```python
from build123d import *

# Parameters (mm, degrees)
SKETCH_1_R      = 4
SKETCH_1_R_2    = 2
EXTRUDE_1_DEPTH = 2
SKETCH_2_R      = 4
SKETCH_2_R_2    = 2
EXTRUDE_2_DEPTH = 2
FILLET_1_R      = 2


with BuildPart() as part:
    # 草图1 → 凸台-拉伸1 (new body)
    with BuildSketch(Plane(origin=(0, 0, 0), x_dir=(1, 0, 0), z_dir=(0, 1, 0))):
        with BuildLine():
            Line((-11.25, 12.5), (11.25, 12.5))
            ThreePointArc((11.25, 12.5), (23.75, 0), (11.25, -12.5))
            Line((11.25, -12.5), (-11.25, -12.5))
            Line((-11.25, -12.5), (-11.25, 12.5))
        make_face()
        with Locations((11.25, 0)):
            Circle(SKETCH_1_R, mode=Mode.SUBTRACT)
        with Locations((18.25, 0)):
            Circle(SKETCH_1_R_2, mode=Mode.SUBTRACT)
        with Locations((11.25, -7)):
            Circle(SKETCH_1_R_2, mode=Mode.SUBTRACT)
        with Locations((4.25, 0)):
            Circle(SKETCH_1_R_2, mode=Mode.SUBTRACT)
        with Locations((11.25, 7)):
            Circle(SKETCH_1_R_2, mode=Mode.SUBTRACT)
    extrude(amount=EXTRUDE_1_DEPTH)

    # 草图2 → 凸台-拉伸2 (add)
    with BuildSketch(Plane.ZY.offset(11.25)):
        with BuildLine():
            Line((-12.5, 0), (12.5, 0))
            Line((12.5, 0), (12.5, 12.5))
            ThreePointArc((12.5, 12.5), (0, 25), (-12.5, 12.5))
            Line((-12.5, 12.5), (-12.5, 0))
        make_face()
        with Locations((0, 12.5)):
            Circle(SKETCH_2_R, mode=Mode.SUBTRACT)
        with Locations((0, 19.5)):
            Circle(SKETCH_2_R_2, mode=Mode.SUBTRACT)
        with Locations((7, 12.5)):
            Circle(SKETCH_2_R_2, mode=Mode.SUBTRACT)
        with Locations((0, 5.5)):
            Circle(SKETCH_2_R_2, mode=Mode.SUBTRACT)
        with Locations((-7, 12.5)):
            Circle(SKETCH_2_R_2, mode=Mode.SUBTRACT)
    extrude(amount=-EXTRUDE_2_DEPTH)

    # 圆角1
    fillet_1_edges = [part.edges().sort_by_distance(p)[0] for p in [
        (-11.25, 0, 0),
    ]]
    fillet(fillet_1_edges, radius=FILLET_1_R)


solid = part.part
```
Check sheet for the modelled part. Datum: model origin and axes. Units: mm. A direction names the side the tool comes from. Coordinates: 2 decimals unless noted, no trailing zeros. Order: outer loops, then holes, each group sorted by start corner. A loop starts at its lowest first (then second) coordinate and runs counter-clockwise, first axis right, second up. Notation, with made-up numbers: M 57,17 L 113,17 A12 ccw 113,29 Z; hole C 46.25,44.25 d4. An arc over 180 degrees is marked long. Write each question's results on one line, items separated by ' | '. Start each with the question number.
1. Cross-section at D-D on z = 9.5. Record the cut outline in (x, y), and give its area (3 significant figures).
2. Mould release check, pull along Y, two halves, no side actions. Record for faces 1 (the face through (-10.65, 0.57, -0.18)), 2 (the face through (9.252, 0.986, 6.912)), 3 (the face through (-10, 25, 0)), 4 (the face through (-10.264, 16.466, -0.521)): +Y half, -Y half, draft (parallel to the pull), parting line (faces both ways), or undercut.
3. Go/stop test with flat-tipped pins: P1, Ø6.5, axis at x = 11.25, z = -7, coming from the +Y side; P2, Ø1, axis at y = 14, z = 10, coming from the +X side; P3, Ø5, axis at x = -7, z = -4, coming from the +Y side. Record where each tip stops, or that it passes through.
4. Access from +Z, -Z, +X, -X, +Y, -Y to the whole of each face (thin tool, end or side, straight path). Record for faces 5 (the face through (4, 2, -3)), 6 (the face through (-2.4, 1.6, 12.5)).
5. Cross-section at A-A on x = 4.25. Record the cut outline in (y, z), and give its area (3 significant figures).
6. Cross-section at C-C on z = 0. State how many separate pieces and enclosed holes the cut face has, and give its area (3 significant figures).
7. Cross-section at B-B on y = 5.5. Record the cut outline in (x, z).
8. Material ranges on probe 1 along Z at (x, y) = (11.25, 0.6); probe 2 along X at (y, z) = (0.6, 0); probe 3 along Y at (x, z) = (-10.35, 0), recorded low to high.
Checks:
1) outline: M -11.25,2 A2 ccw -9.25,0 L 19.37,0 L 19.37,2 L -9.25,2 L -9.25,20.62 L -11.25,20.62 Z | area: 97.6 mm²
2) face 1: -Y half | face 2: draft | face 3: +Y half | face 4: undercut
3) P1: stops at y = 2 | P2: stops at x = -9.25 | P3: stops at y = 24.66
4) face 5: +Z, -Z, +X, +Y | face 6: +Z, +X, -X, +Y, -Y
5) outline: M 0,-12.5 L 2,-12.5 L 2,-2 L 0,-2 Z; M 0,2 L 2,2 L 2,12.5 L 0,12.5 Z | area: 42.0 mm²
6) separate pieces: 7 | enclosed holes: 0 | area: 51.1 mm²
7) outline: M -11.25,-12.5 L -9.25,-12.5 L -9.25,-2 L -11.25,-2 Z; M -11.25,2 L -9.25,2 L -9.25,12.5 L -11.25,12.5 Z
8) probe 1: z = -12.5 to -9, -5 to -4, 4 to 5, 9 to 12.5 | probe 2: x = -10.68 to 2.25, 6.25 to 7.25, 15.25 to 16.25, 20.25 to 23.75 | probe 3: y = 0.33 to 3.5, 7.5 to 8.5, 16.5 to 17.5, 21.5 to 25
